Can you work these out from the drawing? Everything is in mm from the part's minimum corner. A direction names the side the tool comes from. Round coordinates to 2 decimals unless told otherwise and drop trailing zeros. Loops run counter-clockwise (first coordinate to the right, second up) from the corner with the lowest first, then second, coordinate; pieces in that order, holes last. Notation, with made-up numbers: (-10, -27) - (25, -27) arc R20 cw to (25, -5) - close; hole circle Ø9 at (55.5, 64). An arc over 180 degrees is marked (long way). Answer as CSV lines item,"result". Start each with the question number.
1) Suppose I cut it at C-C, the plane x = 1.5. Write out the boundary of the cut face in (y, z).
2) Which directions (+Z, -Z, +X, -X, +Y, -Y) give clear straight access to the entire face, cutting with the end or side of a thin tool? Please do the marked faces 4 and 5.
3) Suppose I cut it at B-B, the plane z = 1.15. Write out the boundary of the cut face in (x, y).
4) I'm going to push flat-ended pins straight in: pin 1 Ø0.8 at (x, y) = (6.5, 15.5) entering from +Z; pin 2 Ø0.7 at (x, z) = (3, 1) entering from +Y; pin 3 Ø0.8 at (x, y) = (1.5, 15.5) entering from -Z. Where does each tip first touch, or does it pass through?
5) Please list where these lines run through material, in increasing order: line 1 along Z through (x, y) = (2, 16); line 2 along X through (y, z) = (14, 0.2); line 3 along Y through (x, z) = (6.25, 1).
6) Suppose I cut it at A-A, the plane y = 12.5. Write out the boundary of the cut face in (x, z).
7) We'd pull the mould along Z, two halves only. Please class the marked faces 1, 2 and 3: pulls with the +Z half, pulls with the -Z half, needs draft (parallel to the pull), parting line crosses it, or undercut.
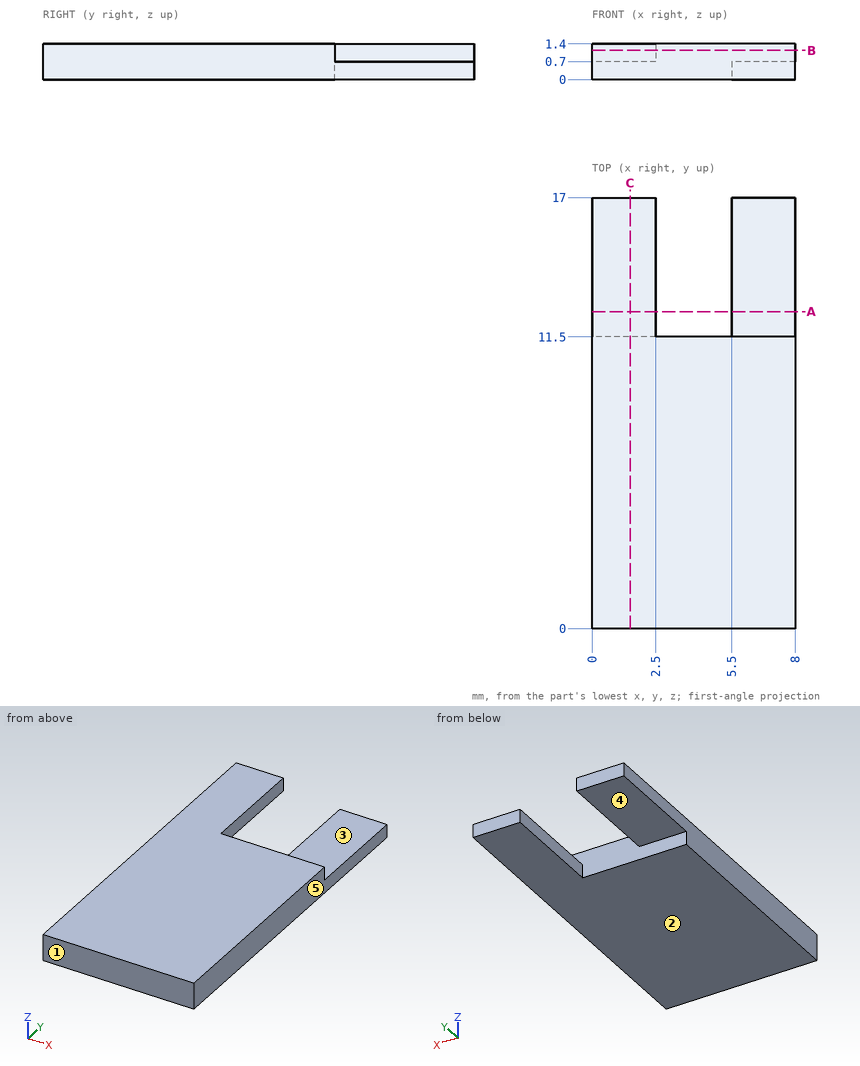
Filled sheet:
1,outline,"(0, 0) - (11.5, 0) - (11.5, 0.7) - (17, 0.7) - (17, 1.4) - (0, 1.4) - close"
2,face 4,"-Z, -X, +Y"
2,face 5,"+Z, -Z, +X, +Y, -Y"
3,outline,"(0, 0) - (8, 0) - (8, 11.5) - (2.5, 11.5) - (2.5, 17) - (0, 17) - close"
4,pin 1,"z = 0.7"
4,pin 2,"y = 11.5"
4,pin 3,"z = 0.7"
5,line 1,"0.7 to 1.4"
5,line 2,"5.5 to 8"
5,line 3,"0 to 11.5"
6,outline,"(0, 0.7) - (2.5, 0.7) - (2.5, 1.4) - (0, 1.4) - close; (5.5, 0) - (8, 0) - (8, 0.7) - (5.5, 0.7) - close"
7,face 1,"needs draft"
7,face 2,"pulls with the -Z half"
7,face 3,"pulls with the +Z half"
